from build123d import *

# Parameters (mm, degrees)
SKETCH1_R           = 0.75
BOSS_EXTRUDE1_DEPTH = 4
BOSS_EXTRUDE2_START = 4.2
SKETCH2_R           = 1.5
BOSS_EXTRUDE2_DEPTH = 4.2


with BuildPart() as part:
    # Sketch1 → Boss-Extrude1 (new body)
    with BuildSketch(Plane(origin=(0, 0, 0), x_dir=(0, 0, -1), z_dir=(1, 0, 0))):
        with BuildLine():
            Line((48.989794856, 11.5), (23.130680142, 11.5))
            ThreePointArc((23.130680142, 11.5), (7.154143168, 13.591545205), (-1.5, 0))
            ThreePointArc((-1.5, 0), (0, -1.5), (1.5, 0))
            ThreePointArc((1.5, 0), (8.898176779, 11.08256392), (21.970537173, 8.5))
            Line((21.970537173, 8.5), (48.989794856, 8.5))
            ThreePointArc((48.989794856, 8.5), (50.489794856, 10), (48.989794856, 11.5))
        make_face()
        with Locations((48.989794856, 10)):
            Circle(SKETCH1_R, mode=Mode.SUBTRACT)
    extrude(amount=BOSS_EXTRUDE1_DEPTH)

    # Sketch2 → Boss-Extrude2 (add)
    with BuildSketch(Plane.ZY.offset(BOSS_EXTRUDE2_START)):
        Circle(SKETCH2_R)
    extrude(amount=-BOSS_EXTRUDE2_DEPTH)


solid = part.part
Geometry: final body of the model. Coordinates: model frame, mm. A direction names the side the tool comes from. Round coordinates to 2 decimals unless told otherwise and drop trailing zeros. Loops run counter-clockwise (first coordinate to the right, second up) from the corner with the lowest first, then second, coordinate; pieces in that order, holes last. Notation, with made-up numbers: (67.5, -21.5) -> (92.5, -21.5) arc R20 cw to (92.5, 2.5) -> close; hole circle Ø10 at (28, 71). An arc over 180 degrees is marked (long way). One line per question, with ' | ' between items. Start each with the question number.
1. Line query: line 1 along Y through (x, z) = (0.75, -24.5); line 2 along X through (y, z) = (11.75, -8); line 3 along Z through (x, y) = (2.75, 9.75). Output: solid intervals per line, ascending. Write a range as [from, to].
2. Section A-A on x = 2.25. Output: boundary loops of the cut face in (y, z), and give its area (3 significant figures).
3. Section B-B on y = 10. Output: boundary loops of the cut face in (x, z), and give its area (3 significant figures).
4. Section C-C on z = 0. Output: boundary loops of the cut face in (x, y), and give its area (3 significant figures).
5. Mould query, pull axis Z, two halves, no side actions, for faces 1 (the face through (1.97, 13.69, -7.37)), 2 (the face through (2, 8.5, -35)), 3 (the face through (2, 11, -8.7)), 4 (the face through (1.97, 9.97, -50.49)). Classes: pulls with the +Z half, pulls with the -Z half, needs draft (parallel to the pull), parting line crosses it, or undercut.
6. Contact query for flat-ended pins moving along their axis: pin 1 (1 mm diameter, centred on x = 3, z = -45, fed in from -Y); pin 2 (1.2 mm diameter, centred on y = 10, z = -48.99, fed in from -X); pin 3 (4.5 mm diameter, centred on x = 2.5, z = -41, fed in from +Y). Output: stop coordinate, or through.
7. Set-up query: faces 5 (the face through (4, 10, -21)), 6 (the face through (-1.069, -1.464, -0.325)), 7 (the face through (2, 11.5, -36)). Return all of +Z, -Z, +X, -X, +Y, -Y with unobstructed straight access to the full face (end or side cutting, diameter ignored); none if empty.
8. Section D-D on x = -1.5. Output: boundary loops of the cut face in (y, z).
Returned:
1) line 1: y = [8.5, 11.5] | line 2: x = [0, 4] | line 3: z = [-50.47, -49.7], [-48.28, -20.5], [-6.5, -2.1]
2) outline: (0, -1.5) arc R12 cw to (8.5, -21.97) -> (8.5, -48.99) arc R1.5 ccw to (11.5, -48.99) -> (11.5, -23.13) arc R15 ccw to (0, 1.5) arc R1.5 ccw to start; hole circle Ø1.5 at (10, -48.99) | area: 178 mm2
3) outline: (0, -50.49) -> (4, -50.49) -> (4, -49.74) -> (0, -49.74) -> close; (0, -48.24) -> (4, -48.24) -> (4, -20.13) -> (0, -20.13) -> close; (0, -6.87) -> (4, -6.87) -> (4, -2.32) -> (0, -2.32) -> close | area: 134 mm2
4) outline: (-4.2, -1.5) -> (4, -1.5) -> (4, 6.54) -> (0, 6.54) -> (0, 1.5) -> (-4.2, 1.5) -> close | area: 44.8 mm2
5) face 1: parting line crosses it | face 2: needs draft | face 3: undercut | face 4: pulls with the -Z half
6) pin 1: stops at y = 8.5 | pin 2: passes through | pin 3: stops at y = 11.5
7) face 5: +Z, -Z, +X, +Y, -Y | face 6: -X | face 7: -Z, +X, -X, +Y
8) outline: circle Ø3 at (0, 0)
